```python
from build123d import *

# Parameters (mm, degrees)
F1_DEPTH = 25.4
F2_SIZE  = 1.27
F3_R     = 5.08
F4_SIZE  = 1.27


with BuildPart() as f1:
    # F0 (on Top) → F1 (new body)
    with BuildSketch(Plane.XY):
        Polygon((13.728917, 33.325016), (0, 0), (89.838997, 0), (76.11008, 33.325016), align=None)
    extrude(amount=F1_DEPTH)

    # F2
    f2_edges = [f1.edges().sort_by_distance(p)[0] for p in [
        (6.864458, 16.662508, 25.4),
        (6.864458, 16.662508, 0),
        (82.974538, 16.662508, 25.4),
        (82.974538, 16.662508, 0),
    ]]
    chamfer(f2_edges, length=F2_SIZE)

    # F3
    f3_edges = [f1.edges().sort_by_distance(p)[0] for p in [
        (44.919498, 0, 0),
        (44.919498, 0, 25.4),
    ]]
    fillet(f3_edges, radius=F3_R)

    # F4
    f4_edges = [f1.edges().sort_by_distance(p)[0] for p in [
        (44.919498, 33.325016, 25.4),
        (44.919498, 33.325016, 0),
    ]]
    chamfer(f4_edges, length=F4_SIZE)


solid = f1.part
```
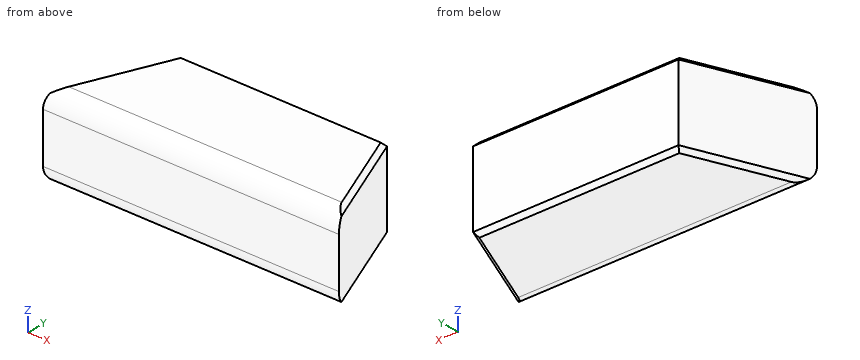
Source: CAD feature listing. Evaluate the final solid. Frame: model axes, mm. Round coordinates to 2 decimals unless told otherwise and drop trailing zeros. Write each loop counter-clockwise with the first axis right and the second up, starting at its lowest first coordinate (ties: lowest second). Pieces come first, ordered by that corner, then holes. Notation, with made-up numbers: M -6.5,73.5 L 4.5,73.5 A32 ccw 4.5,101.5 Z; hole C 17,52.5 d4. An arc over 180 degrees is marked long. Use CSV: the item, a comma, the result in double quotes. Start each with the question number.
Q1. Cut plane C-C on z = 7.25. Output: boundary loops of the cut face in (x, y), plus the area to 3 significant figures.
Q2. Cut plane D-D on z = 3.5. Output: boundary loops of the cut face in (x, y), plus the area to 3 significant figures.
Q3. Cut plane A-A on x = 82.5. Output: boundary loops of the cut face in (y, z), plus the area to 3 significant figures.
Q4. First-contact query: P1, Ø1.5, axis at y = 29, z = 7.5, coming from the +X side; P2, Ø10, axis at y = 19, z = 22, coming from the +X side; P3, Ø8, axis at y = 24.5, z = 4.5, coming from the -X side. Flat tips, straight axial feed; report the tip coordinate or a pass-through.
Q5. Cut plane B-B on y = 18.5. Output: boundary loops of the cut face in (x, z) (3 decimals), plus the area to 3 significant figures.
Q6. Line query: line 1 (X direction, y = 18, z = 22.5); line 2 (X direction, y = 28, z = 24.5); line 3 (Z direction, x = 43, y = 4.5). Output: solid intervals per line, ascending. Write a range as from..to.
Results found:
1,outline,"M 0,0 L 89.84,0 L 76.11,33.33 L 13.73,33.33 Z"
1,area,"2,540 mm^2"
2,outline,"M 0.1,0.25 L 89.74,0.25 L 76.11,33.33 L 13.73,33.33 Z"
2,area,"2,510 mm^2"
3,outline,"M 0,5.08 A5.08 ccw 5.08,0 L 14.48,0 L 17.81,1.27 L 17.81,24.13 L 14.48,25.4 L 5.08,25.4 A5.08 ccw 0,20.32 Z"
3,area,"437 mm^2"
4,P1,"x = 78.2"
4,P2,"x = 84.07"
4,P3,"x = 8.45"
5,outline,"M 7.621,1.27 L 8.995,0 L 80.844,0 L 82.218,1.27 L 82.218,24.13 L 80.844,25.4 L 8.995,25.4 L 7.621,24.13 Z"
5,area,"1,890 mm^2"
6,line 1,"7.42..82.42"
6,line 2,"11.94..77.9"
6,line 3,"0.03..25.37"
